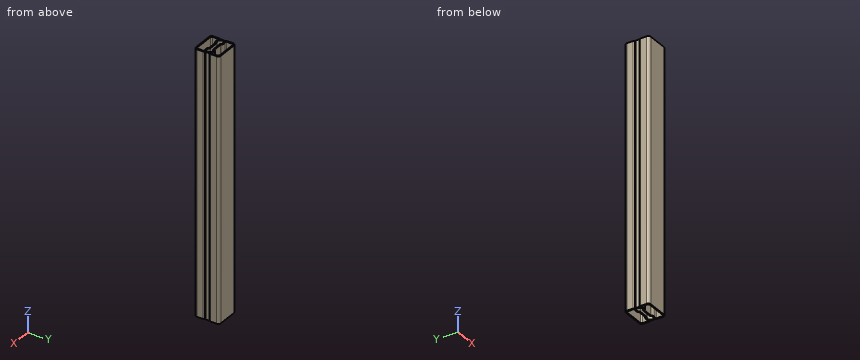
```python
from build123d import *

# Parameters (mm, degrees)
BOSS_EXTRUDE1_DEPTH = 266.7


with BuildPart() as part:
    # Sketch1 → Boss-Extrude1 (new body)
    with BuildSketch(Plane.XY):
        with BuildLine():
            Line((12.7, 3.904831807), (12.7, 10.16))
            ThreePointArc((12.7, 10.16), (11.956051224, 11.956051224), (10.16, 12.7))
            Line((10.16, 12.7), (-10.16, 12.7))
            ThreePointArc((-10.16, 12.7), (-11.956051224, 11.956051224), (-12.7, 10.16))
            Line((-12.7, 10.16), (-12.7, 3.904831807))
            ThreePointArc((-12.7, 3.904831807), (-12.511460601, 3.078521934), (-11.983162199, 2.415773182))
            ThreePointArc((-11.983162199, 2.415773182), (-11.763134535, 2.073265365), (-11.796313868, 1.667527878))
            ThreePointArc((-11.796313868, 1.667527878), (-12.1412, 0), (-11.796313868, -1.667527878))
            ThreePointArc((-11.796313868, -1.667527878), (-11.763134535, -2.073265365), (-11.983162199, -2.415773182))
            ThreePointArc((-11.983162199, -2.415773182), (-12.511460601, -3.078521934), (-12.7, -3.904831807))
            Line((-12.7, -3.904831807), (-12.7, -10.16))
            ThreePointArc((-12.7, -10.16), (-11.956051224, -11.956051224), (-10.16, -12.7))
            Line((-10.16, -12.7), (10.16, -12.7))
            ThreePointArc((10.16, -12.7), (11.956051224, -11.956051224), (12.7, -10.16))
            Line((12.7, -10.16), (12.7, -3.904831807))
            ThreePointArc((12.7, -3.904831807), (12.511460601, -3.078521934), (11.983162199, -2.415773182))
            ThreePointArc((11.983162199, -2.415773182), (11.763134535, -2.073265365), (11.796313868, -1.667527878))
            ThreePointArc((11.796313868, -1.667527878), (12.1412, 0), (11.796313868, 1.667527878))
            ThreePointArc((11.796313868, 1.667527878), (11.763134535, 2.073265365), (11.983162199, 2.415773182))
            ThreePointArc((11.983162199, 2.415773182), (12.511460601, 3.078521934), (12.7, 3.904831807))
        make_face()
        with BuildLine():
            Line((4.467104451, -1.46685), (-4.467104451, -1.46685))
            ThreePointArc((-4.467104451, -1.46685), (-5.208770649, -1.617154514), (-5.833401911, -2.04435))
            ThreePointArc((-5.833401911, -2.04435), (-10.8712, 0), (-5.833401911, 2.04435))
            ThreePointArc((-5.833401911, 2.04435), (-5.208770649, 1.617154514), (-4.467104451, 1.46685))
            Line((-4.467104451, 1.46685), (4.467104451, 1.46685))
            ThreePointArc((4.467104451, 1.46685), (5.208770649, 1.617154514), (5.833401911, 2.04435))
            ThreePointArc((5.833401911, 2.04435), (10.8712, 0), (5.833401911, -2.04435))
            ThreePointArc((5.833401911, -2.04435), (5.208770649, -1.617154514), (4.467104451, -1.46685))
        make_face(mode=Mode.SUBTRACT)
        with BuildLine():
            Line((11.43, 10.16), (11.43, 3.904831807))
            ThreePointArc((11.43, 3.904831807), (11.082315158, 3.338550075), (10.42, 3.392386688))
            ThreePointArc((10.42, 3.392386688), (7.584682807, 4.188867833), (4.922536938, 2.92935))
            ThreePointArc((4.922536938, 2.92935), (4.714326517, 2.786951505), (4.467104451, 2.73685))
            Line((4.467104451, 2.73685), (-4.467104451, 2.73685))
            ThreePointArc((-4.467104451, 2.73685), (-4.714326517, 2.786951505), (-4.922536938, 2.92935))
            ThreePointArc((-4.922536938, 2.92935), (-7.584682807, 4.188867833), (-10.42, 3.392386688))
            ThreePointArc((-10.42, 3.392386688), (-11.082315158, 3.338550075), (-11.43, 3.904831807))
            Line((-11.43, 3.904831807), (-11.43, 10.16))
            ThreePointArc((-11.43, 10.16), (-11.058025612, 11.058025612), (-10.16, 11.43))
            Line((-10.16, 11.43), (10.16, 11.43))
            ThreePointArc((10.16, 11.43), (11.058025612, 11.058025612), (11.43, 10.16))
        make_face(mode=Mode.SUBTRACT)
        with BuildLine():
            Line((11.43, -3.904831807), (11.43, -10.16))
            ThreePointArc((11.43, -10.16), (11.058025612, -11.058025612), (10.16, -11.43))
            Line((10.16, -11.43), (-10.16, -11.43))
            ThreePointArc((-10.16, -11.43), (-11.058025612, -11.058025612), (-11.43, -10.16))
            Line((-11.43, -10.16), (-11.43, -3.904831807))
            ThreePointArc((-11.43, -3.904831807), (-11.082315158, -3.338550075), (-10.42, -3.392386688))
            ThreePointArc((-10.42, -3.392386688), (-7.584682807, -4.188867833), (-4.922536938, -2.92935))
            ThreePointArc((-4.922536938, -2.92935), (-4.714326517, -2.786951505), (-4.467104451, -2.73685))
            Line((-4.467104451, -2.73685), (4.467104451, -2.73685))
            ThreePointArc((4.467104451, -2.73685), (4.714326517, -2.786951505), (4.922536938, -2.92935))
            ThreePointArc((4.922536938, -2.92935), (7.584682807, -4.188867833), (10.42, -3.392386688))
            ThreePointArc((10.42, -3.392386688), (11.082315158, -3.338550075), (11.43, -3.904831807))
        make_face(mode=Mode.SUBTRACT)
    extrude(amount=-BOSS_EXTRUDE1_DEPTH)


solid = part.part
```
Design review of the part built by this model. Coordinates are the model's own, in mm. Coordinates: 2 decimals unless noted, no trailing zeros. Write each loop counter-clockwise with the first axis right and the second up, starting at its lowest first coordinate (ties: lowest second). Pieces come first, ordered by that corner, then holes.
1) To check wall thickness, follow L1, parallel to Y at x = -1.75, z = -181; L2, parallel to Y at x = -8, z = -59; L3, parallel to X at y = -0.5, z = -21.5. State the ranges of each line that lie inside material, in increasing order.
2) Add section B-B (z = -203.5). State how many separate pieces and enclosed holes the cut face has, plus the area to 3 significant figures.
3) Add section A-A (y = 7.5). Write out the cut boundary in (x, z).
Check result:
1. L1: y = -12.7 to -11.43, -2.74 to -1.47, 1.47 to 2.74, 11.43 to 12.7
1. L2: y = -12.7 to -11.43, -4.2 to -2.93, 2.93 to 4.2, 11.43 to 12.7
1. L3: x = -12.11 to -10.83, 10.83 to 12.11
2. separate pieces: 1
2. enclosed holes: 3
2. area: 178 mm2
3. outline: (-12.7, -266.7) - (-11.43, -266.7) - (-11.43, 0) - (-12.7, 0) - close; (11.43, -266.7) - (12.7, -266.7) - (12.7, 0) - (11.43, 0) - close
